from build123d import *

# Parameters (mm, degrees)
SKETCH1_W           = 66
SKETCH1_H           = 50
SKETCH1_R           = 1.65
BOSS_EXTRUDE1_DEPTH = 5
SKETCH2_W           = 36
SKETCH2_H           = 36
BOSS_EXTRUDE2_DEPTH = 1.8
CUT_EXTRUDE1_REACH  = 62.117
SKETCH3_W           = 5
SKETCH3_H           = 3.2
FILLET1_R           = 1


with BuildPart() as part:
    # Sketch1 → Boss-Extrude1 (new body)
    with BuildSketch(Plane(origin=(0, 0, 0), x_dir=(1, 0, 0), z_dir=(0, 1, 0))):
        Rectangle(SKETCH1_W, SKETCH1_H)
        with Locations(Location((-28, 20.6, 0), (0, 0, 270))):
            Circle(SKETCH1_R, mode=Mode.SUBTRACT)
        with Locations(Location((28, 20.6, 0), (0, 0, 270))):
            Circle(SKETCH1_R, mode=Mode.SUBTRACT)
        with Locations(Location((-28, -20.6, 0), (0, 0, 270))):
            Circle(SKETCH1_R, mode=Mode.SUBTRACT)
        with Locations(Location((28, -20.6, 0), (0, 0, 270))):
            Circle(SKETCH1_R, mode=Mode.SUBTRACT)
        Polygon((20.1, -20.1), (20.1, 21.1), (18.1, 21.1), (18.1, 20.1), (-18.1, 20.1), (-18.1, 21.1), (-20.1, 21.1), (-20.1, -20.1), align=None, mode=Mode.SUBTRACT)
    extrude(amount=BOSS_EXTRUDE1_DEPTH)

    # Sketch2 → Boss-Extrude2 (add)
    with BuildSketch(Plane(origin=(0, 5, 0), x_dir=(1, 0, 0), z_dir=(0, 1, 0))):
        Polygon((-20.1, 21.1), (-20.1, -20.1), (20.1, -20.1), (20.1, 21.1), (18.1, 21.1), (18.1, 20.1), (-18.1, 20.1), (-18.1, 21.1), align=None)
        Rectangle(SKETCH2_W, SKETCH2_H, mode=Mode.SUBTRACT)
    extrude(amount=-BOSS_EXTRUDE2_DEPTH)

    # Sketch3 → Cut-Extrude1 (cut, up to next)
    with BuildSketch(Plane.XY.offset(25), mode=Mode.PRIVATE) as cut_extrude1_sk1:
        with Locations((-17.6, 1.6)):
            Rectangle(SKETCH3_W, SKETCH3_H)
    cut_extrude1_tool1 = extrude(cut_extrude1_sk1.sketch, amount=-CUT_EXTRUDE1_REACH, mode=Mode.PRIVATE) & part.part
    # Sketch3 → Cut-Extrude1 (cut, up to next)
    with BuildSketch(Plane.XY.offset(25), mode=Mode.PRIVATE) as cut_extrude1_sk2:
        with Locations((17.6, 1.6)):
            Rectangle(SKETCH3_W, SKETCH3_H)
    cut_extrude1_tool2 = extrude(cut_extrude1_sk2.sketch, amount=-CUT_EXTRUDE1_REACH, mode=Mode.PRIVATE) & part.part
    add(cut_extrude1_tool1.solids().sort_by_distance((-17.6, 1.6, 25))[0], mode=Mode.SUBTRACT)
    add(cut_extrude1_tool2.solids().sort_by_distance((17.6, 1.6, 25))[0], mode=Mode.SUBTRACT)

    # Fillet1
    fillet1_edges = [part.edges().sort_by_distance(p)[0] for p in [
        (-18, 4.1, 18),
        (18, 4.1, 18),
        (18, 4.1, -18),
        (-18, 4.1, -18),
        (-20.1, 1.6, -21.1),
        (-18.1, 1.6, -21.1),
        (18.1, 1.6, -21.1),
        (20.1, 1.6, -21.1),
    ]]
    fillet(fillet1_edges, radius=FILLET1_R - 0.0001)  # a hair under: the kernel refuses the full size


solid = part.part
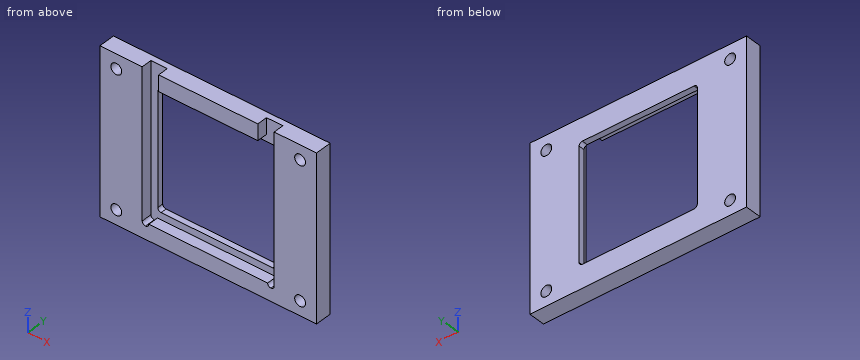
Input: part model. Units: mm. Frame: model coordinates. Round coordinates to 2 decimals unless told otherwise and drop trailing zeros. Loops run counter-clockwise (first coordinate to the right, second up) from the corner with the lowest first, then second, coordinate; pieces in that order, holes last. Notation, with made-up numbers: (-7.5, 55) -> (28.5, 55) arc R28 cw to (28.5, 89) -> close; hole circle Ø3 at (71, 43.5). An arc over 180 degrees is marked (long way). Answer as a JSON object with one key per item and string values. Group by question number.
1) Section query D-D on x = -28. Output: boundary loops of the cut face in (y, z), plus the area to 3 significant figures.
2) Section query C-C on z = -9. Output: boundary loops of the cut face in (x, y), plus the area to 3 significant figures.
3) Section query B-B on x = -7. Output: boundary loops of the cut face in (y, z).
4) Section query A-A on y = 2.3. State how many separate pieces and enclosed holes the cut face has, plus the area to 3 significant figures.
5) Ray query, L1, parallel to X at y = 3.1, z = 20.6; L2, parallel to Z at x = 14.5, y = 0.5; L3, parallel to X at y = 3.7, z = -20.6. Return the intervals inside material, ascending.
Reply:
{
 "1": {"outline": "(0, -25) -> (5, -25) -> (5, -22.25) -> (0, -22.25) -> close; (0, -18.95) -> (5, -18.95) -> (5, 18.95) -> (0, 18.95) -> close; (0, 22.25) -> (5, 22.25) -> (5, 25) -> (0, 25) -> close", "area": "217 mm2"},
 "2": {"outline": "(-33, 0) -> (-20.1, 0) -> (-20.1, 3.2) -> (-18, 3.2) -> (-18, 5) -> (-33, 5) -> close; (18, 3.2) -> (20.1, 3.2) -> (20.1, 0) -> (33, 0) -> (33, 5) -> (18, 5) -> close", "area": "137 mm2"},
 "3": {"outline": "(0, -25) -> (5, -25) -> (5, -18) -> (3.2, -18) -> (3.2, -20.1) -> (0, -20.1) -> close; (0, 20.1) -> (3.2, 20.1) -> (3.2, 18) -> (5, 18) -> (5, 25) -> (0, 25) -> close"},
 "4": {"separate pieces": "2", "enclosed holes": "4", "area": "1,600 mm2"},
 "5": {"L1": "x = -33 to -29.65, -26.35 to -20.1, -15.1 to 15.1, 20.1 to 26.35, 29.65 to 33", "L2": "z = -25 to -20.1, 20.1 to 25", "L3": "x = -33 to -29.65, -26.35 to 26.35, 29.65 to 33"}
}
